```python
from build123d import *

# Parameters (mm, degrees)
SKETCH1_R               = 4
BOSS_EXTRUDE1_DEPTH     = 30
BOSS_EXTRUDE1_2_DEPTH   = 30
SKETCH2_W               = 86.738485283
SKETCH2_H               = 68.254231625
BOSS_EXTRUDE2_DEPTH     = 2
SKETCH4_W               = 70.255349131
SKETCH4_H               = 2
CUT_EXTRUDE_THIN1_DEPTH = 2
SKETCH3_W               = 86.738485283
SKETCH3_H               = 64
BOSS_EXTRUDE3_DEPTH     = 2


with BuildPart() as part:
    # Sketch1 → Boss-Extrude1 (new body, symmetric)
    with BuildSketch(Plane.XY):
        with Locations((-25, -30.44)):
            Circle(SKETCH1_R)
    extrude(amount=BOSS_EXTRUDE1_DEPTH, both=True)



with BuildPart() as body_2:
    # Sketch1 → Boss-Extrude1 2 (new body, symmetric)
    with BuildSketch(Plane.XY):
        with Locations((25, -30.44)):
            Circle(SKETCH1_R)
    extrude(amount=BOSS_EXTRUDE1_2_DEPTH, both=True)


with BuildPart() as part_1:
    add(part.part)

    add(body_2.part)  # Boss-Extrude2 merges body 2
    # Sketch2 → Boss-Extrude2 (add)
    with BuildSketch(Plane.XY.offset(30)):
        with Locations((-2.776823357, -7.681992187)):
            Rectangle(SKETCH2_W, SKETCH2_H)
    boss_extrude2 = extrude(amount=BOSS_EXTRUDE2_DEPTH)

    # Sketch4 → Cut-Extrude-Thin1 (cut)
    with BuildSketch(Plane.XY.offset(32)):
        with Locations((-2.776823357, 17.267458724)):
            Rectangle(SKETCH4_W, SKETCH4_H)
        with Locations((-2.776823357, 7.267458724)):
            Rectangle(SKETCH4_W, SKETCH4_H)
        with Locations((-2.776823357, -2.732541276)):
            Rectangle(SKETCH4_W, SKETCH4_H)
        with Locations((-2.776823357, -12.732541276)):
            Rectangle(SKETCH4_W, SKETCH4_H)
        with Locations((-2.776823357, -22.732541276)):
            Rectangle(SKETCH4_W, SKETCH4_H)
    cut_extrude_thin1 = extrude(amount=-CUT_EXTRUDE_THIN1_DEPTH, mode=Mode.SUBTRACT)

    # Mirror1: Boss-Extrude2, Cut-Extrude-Thin1 across plane
    add(boss_extrude2.mirror(Plane.XY))
    add(cut_extrude_thin1.mirror(Plane.XY), mode=Mode.SUBTRACT)

    # Sketch3 → Boss-Extrude3 (add)
    with BuildSketch(Plane.XZ.offset(41.809107999)):
        with Locations((-2.776823357, 0)):
            Rectangle(SKETCH3_W, SKETCH3_H)
    extrude(amount=BOSS_EXTRUDE3_DEPTH)


solid = part_1.part
```
Verification items for the finished model (mm, model axes). A direction names the side the tool comes from. Round coordinates to 2 decimals unless told otherwise and drop trailing zeros. Order: outer loops, then holes, each group sorted by start corner. A loop starts at its lowest first (then second) coordinate and runs counter-clockwise, first axis right, second up. Notation, with made-up numbers: (-22, 35.5) - (20, 35.5) arc R23 ccw to (20, 68.5) - close; hole circle Ø2 at (-40, -1). An arc over 180 degrees is marked (long way). Use CSV: the item, a comma, the result in double quotes. Start each with the question number.
1) Section check C-C, the plane x = -13.5. State how many separate pieces and enclosed holes the cut face has, plus the area to 3 significant figures.
2) Go/stop test with a flat-tipped pin: P1, Ø5, axis at x = 3.5, z = 2, coming from the +Y side. Record where the tip stops, or that it passes through.
3) Section check A-A, the plane y = 15. Record the cut outline in (x, z), plus the area to 3 significant figures.
4) Section check D-D, the plane y = -30.44. Record the cut outline in (x, z), plus the area to 3 significant figures.
5) Access from +Z, -Z, +X, -X, +Y, -Y to the whole of each face (thin tool, end or side, straight path). Record for faces 1 (the flat face through (-3, -41.809, 0)), 2 (the cylindrical face through (24.133, -34.345, 0.42)), 3 (the flat face through (-37.904, -23, 31)).
6) Thickness scan on L1, parallel to Z at x = 20.5, y = -14; L2, parallel to Y at x = 5, z = -14.5; L3, parallel to Y at x = -28, z = -15.5. Record the ranges inside material, lowest first.
7) Section check B-B, the plane z = 9.5. Record the cut outline in (x, y), plus the area to 3 significant figures.
8) Mould release check, pull along Y, two halves, no side actions. Record for faces 4 (the flat face through (-3, -43.809, 0)), 5 (the flat face through (32.351, -13, -31)), 6 (the flat face through (-37.904, 17, -31)), 7 (the flat face through (-3, 26.445, -31)): +Y half, -Y half, draft (parallel to the pull), parting line (faces both ways), or undercut.
Answers:
1,separate pieces,"11"
1,enclosed holes,"0"
1,area,"361 mm²"
2,P1,"stops at y = -41.81"
3,outline,"(-46.15, -32) - (40.59, -32) - (40.59, -30) - (-46.15, -30) - close; (-46.15, 30) - (40.59, 30) - (40.59, 32) - (-46.15, 32) - close"
3,area,"347 mm²"
4,outline,"(-46.15, -32) - (40.59, -32) - (40.59, -30) - (29, -30) - (29, 30) - (40.59, 30) - (40.59, 32) - (-46.15, 32) - (-46.15, 30) - (-29, 30) - (-29, -30) - (-46.15, -30) - close; hole (-21, -30) - (21, -30) - (21, 30) - (-21, 30) - close"
4,area,"1,310 mm²"
5,face 1,"+X, -X"
5,face 2,"none"
5,face 3,"+Z, -Z"
6,L1,"z = -32 to -30, 30 to 32"
6,L2,"y = -43.81 to -41.81"
6,L3,"y = -43.81 to -41.81, -33.09 to -27.79"
7,outline,"(-46.15, -43.81) - (40.59, -43.81) - (40.59, -41.81) - (-46.15, -41.81) - close; circle Ø8 at (-25, -30.44); circle Ø8 at (25, -30.44)"
7,area,"274 mm²"
8,face 4,"-Y half"
8,face 5,"undercut"
8,face 6,"undercut"
8,face 7,"+Y half"
